CAD build for the part. Positions are in the model's coordinates, mm. A direction names the side the tool comes from. Round coordinates to 2 decimals unless told otherwise and drop trailing zeros. Loops run counter-clockwise (first coordinate to the right, second up) from the corner with the lowest first, then second, coordinate; pieces in that order, holes last. Notation, with made-up numbers: M 86.25,-30 L 113.25,-30 A13 cw 113.25,-18 Z; hole C 77,41 d3. An arc over 180 degrees is marked long. One line per item, written item: value. Start each with the question number.
from build123d import *

# Parameters (mm, degrees)
EXTRUDE_1_DEPTH     = 4
SKETCH_6_W          = 17
SKETCH_6_H          = 35
EXTRUDE_2_DEPTH     = 4
SKETCH_7_W          = 13
SKETCH_7_H          = 24
CUT_EXTRUDE_3_DEPTH = 12.1
SKETCH_8_W          = 4
SKETCH_8_H          = 4
SKETCH_8_R          = 1.175
EXTRUDE_3_DEPTH     = 15
EXTRUDE_4_DEPTH     = 5
SKETCH_10_R         = 1.175
CUT_EXTRUDE_4_DEPTH = 12.7
CUT_EXTRUDE_6_DEPTH = 3
SKETCH_13_R         = 1.25
CUT_EXTRUDE_7_DEPTH = 13


with BuildPart() as part:
    # 草圖1 → 填料-伸長1 (new body)
    with BuildSketch(Plane.XY):
        with BuildLine():
            Line((7.5, 0), (7.5, 58))
            ThreePointArc((7.5, 58), (0, 65.5), (-7.5, 58))
            Line((-7.5, 58), (-7.5, 0))
            Line((-7.5, 0), (7.5, 0))
        make_face()
    extrude(amount=EXTRUDE_1_DEPTH)

    # 草圖6 → 填料-伸長2 (add)
    with BuildSketch(Plane.XY):
        with Locations((0, -17.5)):
            Rectangle(SKETCH_6_W, SKETCH_6_H)
    extrude(amount=EXTRUDE_2_DEPTH)

    # 草圖7 → 除料-伸長3 (cut)
    with BuildSketch(Plane.XY):
        with Locations((0, -18)):
            Rectangle(SKETCH_7_W, SKETCH_7_H)
    extrude(amount=CUT_EXTRUDE_3_DEPTH, mode=Mode.SUBTRACT)

    # 草圖8 → 填料-伸長3 (add)
    with BuildSketch(Plane.XY):
        with Locations((0, -4)):
            Rectangle(SKETCH_8_W, SKETCH_8_H)
        with Locations((0, -4)):
            Circle(SKETCH_8_R, mode=Mode.SUBTRACT)
    extrude(amount=-EXTRUDE_3_DEPTH)

    # 草圖9 → 填料-伸長4 (add)
    with BuildSketch(Plane(origin=(0, -35, 0), x_dir=(1, 0, 0), z_dir=(0, 1, 0))):
        Polygon((-8.5, 0), (-5, 0), (-5, 5), (5, 5), (5, 0), (8.5, 0), (8.5, 15), (-8.5, 15), align=None)
    extrude(amount=EXTRUDE_4_DEPTH)

    # 草圖10 → 除料-伸長4 (cut)
    with BuildSketch(Plane(origin=(0, 0, -15), x_dir=(-1, 0, 0), z_dir=(0, 0, -1))):
        with Locations((0, -32.5)):
            Circle(SKETCH_10_R)
    extrude(amount=-CUT_EXTRUDE_4_DEPTH, mode=Mode.SUBTRACT)

    # 草圖11 → 除料-伸長6 (cut)
    with BuildSketch(Plane(origin=(0, 0, 0), x_dir=(-1, 0, 0), z_dir=(0, 0, -1))):
        with BuildLine():
            Line((5.049815955, 39.60423521), (2.470722118, 21.775887923))
            ThreePointArc((2.470722118, 21.775887923), (0.036377399, 19.816776136), (-2.09239788, 22.10423521))
            Line((-2.09239788, 22.10423521), (-4.950184045, 39.60423521))
            Line((-4.950184045, 39.60423521), (-2.082979546, 57.10423521))
            ThreePointArc((-2.082979546, 57.10423521), (0.200975521, 59.388190276), (2.484930588, 57.10423521))
            Line((2.484930588, 57.10423521), (5.049815955, 39.60423521))
        make_face()
    extrude(amount=-CUT_EXTRUDE_6_DEPTH, mode=Mode.SUBTRACT)

    # 草圖13 → 除料-伸長7 (cut)
    with BuildSketch(Plane(origin=(0, 0, 0), x_dir=(-1, 0, 0), z_dir=(0, 0, -1))):
        with Locations((0.049815955, 39.60423521)):
            Circle(SKETCH_13_R)
    extrude(amount=-CUT_EXTRUDE_7_DEPTH, mode=Mode.SUBTRACT)


solid = part.part
(1) Slice it at B-B, the plane y = -4. List the corners of the cut face in (x, z) (3 decimals), and give its area (4 significant figures).
(2) Slice it at D-D, the plane y = -32.5. List the corners of the cut face in (x, z) (3 decimals), and give its area (4 significant figures).
(3) Mould opens along Z. For faces 1 (the flat face through (0, -34, -15)), 2 (the flat face through (3.537, 48.232, 1.479)), 3 (the flat face through (5, -33, -3)) say: pulls with the +Z half, pulls with the -Z half, needs draft (parallel to the pull), parting line crosses it, or undercut.
(4) Slice it at A-A, the plane z = -2.75. List the corners of the cut face in (x, y) (3 decimals), and give its area (3 significant figures).
(5) Probe L1, parallel to Y at x = 0, z = -12 (3 decimals); L2, parallel to Y at x = 0.5, z = -5.5; L3, parallel to Y at x = 0, z = -4.25 (3 decimals). List the from-to ranges inside material, lowest first.
(6) Slice it at C-C, the plane x = 0. Count the separate pieces of the cut face and the enclosed holes in it, and give its area (3 significant figures).
(7) Which spindle directions (+Z, -Z, +X, -X, +Y, -Y) get a long thin tool onto all of the face, cutting with end or side? Do faces 4 (the flat face through (0, -6, -4)), 5 (the flat face through (0, -2, -7)), 6 (the flat face through (-7.5, 29, 2)), 7 (the cylindrical face through (-0.151, 59.388, 1.479)). Say none if no direction does.
(8) Flat gauge pins, fed straight in: P1, Ø3, axis at x = -0.05, y = 39.6, coming from the +Z side; P2, Ø0.7, axis at x = 0, y = -4.5, coming from the -Z side; P3, Ø1.5, axis at x = -2.5, z = -4, coming from the -Y side; P4, Ø5, axis at x = -1, y = 35.5, coming from the -Z side. Where does each tip first touch, or does it go through?
Check result:
1. outline: M -8.5,0 L -2,0 L -2,-15 L -1.175,-15 L -1.175,0 L 1.175,0 L 1.175,-15 L 2,-15 L 2,0 L 8.5,0 L 8.5,4 L -8.5,4 Z
1. area: 92.75 mm^2
2. outline: M -8.5,-15 L -1.175,-15 L -1.175,-5 L -5,-5 L -5,0 L 5,0 L 5,-5 L 1.175,-5 L 1.175,-15 L 8.5,-15 L 8.5,4 L -8.5,4 Z
2. area: 249.5 mm^2
3. face 1: pulls with the -Z half
3. face 2: needs draft
3. face 3: undercut
4. outline: M -8.5,-35 L -5,-35 L -5,-30 L -8.5,-30 Z; M -2,-6 L 2,-6 L 2,-2 L -2,-2 Z; M 5,-35 L 8.5,-35 L 8.5,-30 L 5,-30 Z; hole C 0,-4 d2.35
4. area: 46.7 mm^2
5. L1: y = -35 to -33.675, -31.325 to -30, -6 to -5.175, -2.825 to -2
5. L2: y = -35 to -33.56, -31.44 to -30, -6 to -5.06, -2.94 to -2
5. L3: y = -6 to -5.175, -2.825 to -2
6. separate pieces: 5
6. enclosed holes: 0
6. area: 236 mm^2
7. face 4: +Z, -Z
7. face 5: -Z, +X, -X, +Y
7. face 6: +Z, -Z, -X, +Y
7. face 7: -Z
8. P1: stops at z = 4
8. P2: stops at z = 0
8. P3: stops at y = -6
8. P4: stops at z = 3
